Model file for the job. Use its own axes, mm. A direction names the side the tool comes from. Coordinates: 2 decimals unless noted, no trailing zeros. Order: outer loops, then holes, each group sorted by start corner. A loop starts at its lowest first (then second) coordinate and runs counter-clockwise, first axis right, second up. Notation, with made-up numbers: (12, 76) -> (65, 76) arc R13 ccw to (65, 99) -> close; hole circle Ø5 at (-10, 7.5). An arc over 180 degrees is marked (long way). Return JSON: item names as keys, results as strings. Group by question number.
1) Flat gauge pins, fed straight in: pin 1 (0.8 mm diameter, centred on y = 1.5, z = 1.5, fed in from +X); pin 2 (10 mm diameter, centred on x = 6, z = 39, fed in from -Y); pin 3 (10 mm diameter, centred on x = -5.5, y = 20, fed in from +Z); pin 4 (1.8 mm diameter, centred on x = -10, y = 14, fed in from -Z). Where does each tip first touch, or does it go through?
2) Cut at D-D (x = 6). Write the cut outline in (y, z).
3) Cut at C-C (y = 14). Write the cut outline in (x, z), and give its area (3 significant figures).
4) Which spindle directions (+Z, -Z, +X, -X, +Y, -Y) get a long thin tool onto all of the face, cutting with end or side? Do faces 1 (the flat face through (9, 23, 59)), 2 (the flat face through (0, 1, 2)), 3 (the flat face through (9, 25, 57)), 4 (the flat face through (3, 19, 8)), 5 (the flat face through (0, 23, 22)). Say none if no direction does.
5) Probe line 1 (Y direction, x = -10, z = 2); line 2 (X direction, y = 15.5, z = 13.5). List the from-to ranges inside material, lowest first.
6) Cut at A-A (x = -10). Write the cut outline in (y, z).
7) Cut at B-B (z = 14). Write the cut outline in (x, y).
Autodesk Inventor part; units mm, degrees
ref_plane "YZ Plane" through (0, 0, 0) normal (1, 0, 0) x (0, 1, 0)
ref_plane "XZ Plane" through (0, 0, 0) normal (0, 1, 0) x (-1, 0, 0)
ref_plane "XY Plane" through (0, 0, 0) normal (0, 0, 1) x (1, 0, 0)
sketch "Sketch1" plane through (0, 0, 0) normal (1, 0, 0) x (0, 1, 0)
  line L0 (0, 0) -> (30, 0)
  line L1 (30, 0) -> (30, 30)
  line L2 (30, 30) -> (0, 30)
  line L3 (0, 30) -> (0, 0)
  line L4 (0, 0) -> (27, 30)
  dimension "d0" = 30
  dimension "d1" = 30
  dimension "d24" = 3
extrude "Extrusion1" add sketch "Sketch1" along normal blind 3 contours L4 L2 L1 L0
sketch "Sketch2" plane through (0, 0, 0) normal (-1, 0, 0) x (0, 0, 1)
  line L0 (30, 0) -> (0, 0)
  line L1 (0, 0) -> (3, 0)
  line L2 (3, 0) -> (3, 30)
  line L3 (3, 30) -> (0, 30)
  line L4 (0, 30) -> (0, 0)
  line L5 (0, 30) -> (30, 30)
  dimension "d4" = 3
extrude "Extrusion2" add sketch "Sketch2" along normal blind 20
sketch "Sketch3" plane through (0, 0, 3) normal (0, 0, 1) x (1, 0, 0)
  circle A0 centre (-10, 14) radius 1.5
  line L0 (0, 30) -> (-20, 30)
  line L1 (0, 0) -> (-20, 0)
  line L2 (-20, 0) -> (-20, 30)
  line L3 (0, 30) -> (0, 0)
  dimension "d7" = 3
  dimension "d8" = 16
  dimension "d10" = 10
  dimension "d11" = 10
extrude "Extrusion3" cut sketch "Sketch3" against normal through all contours A0
sketch "Sketch4" plane through (3, 0, 0) normal (1, 0, 0) x (0, 0, -1)
  line L0 (0, 0) -> (0, 30)
  line L1 (0, 30) -> (-60, 30)
  line L2 (-60, 30) -> (-60, 27)
  line L3 (-60, 27) -> (0, 27)
  line L4 (0, 27) -> (0, 30)
  point P0 (0, 27)
  dimension "d17" = 3
  dimension "d18" = 60
extrude "Extrusion4" add sketch "Sketch4" along normal blind 15 and the other way blind 3
sketch "Sketch5" plane through (3, 27, 0) normal (0, -1, 0) x (1, 0, 0)
  line L0 (15, 60) -> (15, 0)
  line L1 (15, 60) -> (-3, 60)
  line L2 (-3, 60) -> (-3, 57)
  line L3 (-3, 57) -> (15, 57)
  line L4 (15, 57) -> (15, 60)
  line L5 (-3, 30) -> (-3, 60)
  point P0 (-3, 0)
  dimension "d21" = 3
extrude "Extrusion5" add sketch "Sketch5" along normal blind 4
chamfer "Chamfer1" distance 1 angle 45 3 edges at (3, 27, 15) (0, 16.35, 3) (9, 27, 57)
equation "\"d10\" = d11"
properties part number "inside bracket"
Answers below:
{
 "1": {"pin 1": "stops at x = 3", "pin 2": "stops at y = 27", "pin 3": "stops at z = 3.5", "pin 4": "passes through"},
 "2": {"outline": "(23, 57) -> (26, 57) -> (27, 56) -> (27, 0) -> (30, 0) -> (30, 60) -> (23, 60) -> close"},
 "3": {"outline": "(-20, 0) -> (-11.5, 0) -> (-11.5, 3) -> (-20, 3) -> close; (-8.5, 0) -> (3, 0) -> (3, 15.56) -> (0, 15.56) -> (0, 4) -> (-1, 3) -> (-8.5, 3) -> close", "area": "98.2 mm^2"},
 "4": {"face 1": "+Z, +X, -X, -Y", "face 2": "+Z, +X, -Y", "face 3": "+X, -X, -Y", "face 4": "-Z, +X, -Y", "face 5": "+Z, -X, +Y, -Y"},
 "5": {"line 1": "y = 0 to 12.5, 15.5 to 30", "line 2": "x = 0 to 3"},
 "6": {"outline": "(0, 0) -> (12.5, 0) -> (12.5, 3) -> (0, 3) -> close; (15.5, 0) -> (30, 0) -> (30, 3) -> (15.5, 3) -> close"},
 "7": {"outline": "(0, 12.6) -> (3, 12.6) -> (3, 26) -> (4, 27) -> (18, 27) -> (18, 30) -> (0, 30) -> close"}
}
